Part model, mm, in its own coordinate system. A direction names the side the tool comes from. Round coordinates to 2 decimals unless told otherwise and drop trailing zeros.
1) Saw through at A-A on z = 686. Count the separate pieces of the cut face and the enclosed holes in it, and give its area (3 significant figures).
2) Which spindle directions (+Z, -Z, +X, -X, +Y, -Y) get a long thin tool onto all of the face, cutting with end or side? Do faces 1 (the cylindrical face through (6.81, -15.137, 493)), 2 (the flat face through (11, 14, 0)), 3 (the flat face through (52, 20, 493)). Say none if no direction does.
3) Pull direction X, two halves, no side cores. Call faces 4 (the flat face through (28, -20, 493)), 5 (the cylindrical face through (-7.972, -8.594, 493)), 6 (the flat face through (20, 52, 493)), 7 (the cylindrical face through (-15, 6.45, 493)): +X half, -X half, draft (parallel to the pull), parting line (faces both ways), or undercut.
4) Flat gauge pins, fed straight in: pin 1 (7.5 mm diameter, centred on x = 11.5, z = 603, fed in from -Y); pin 2 (5 mm diameter, centred on x = 30, y = -4, fed in from +Z); pin 3 (1 mm diameter, centred on x = 6, z = 274, fed in from -Y); pin 4 (2 mm diameter, centred on x = 32.5, z = 486.5, fed in from +Y). Where does each tip first touch, or does it go through?
5) Drill centre lines: L1, parallel to X at y = 48, z = 777; L2, parallel to Y at x = -2.5, z = 74; L3, parallel to X at y = 14.5, z = 181.5. Where is each one in solid material? Low to high.
```python
from build123d import *

# Parameters (mm, degrees)
SKETCH_1_R      = 3.4
SKETCH_1_R_2    = 4.3
EXTRUDE_1_DEPTH = 1000


with BuildPart() as part:
    # Эскиз1 → Бобышка-Вытянуть1 (new body)
    with BuildSketch(Plane.XY):
        with BuildLine():
            Line((-20, 47.35), (-20, 60))
            Line((-20, 60), (-7.35, 60))
            Line((-7.35, 60), (-4.1, 60))
            Line((-4.1, 60), (-4.1, 56.4))
            Line((-4.1, 56.4), (-7.35, 56.4))
            Line((-7.35, 56.4), (-7.35, 49.4))
            ThreePointArc((-7.35, 49.4), (0, 45.918928476), (7.35, 49.4))
            Line((7.35, 49.4), (7.35, 56.4))
            Line((7.35, 56.4), (4.1, 56.4))
            Line((4.1, 56.4), (4.1, 60))
            Line((4.1, 60), (7.35, 60))
            Line((7.35, 60), (20, 60))
            Line((20, 60), (20, 47.35))
            Line((20, 47.35), (20, 44.1))
            Line((20, 44.1), (16.4, 44.1))
            Line((16.4, 44.1), (16.4, 47.35))
            Line((16.4, 47.35), (9.4, 47.35))
            ThreePointArc((9.4, 47.35), (5.918928476, 40), (9.4, 32.65))
            Line((9.4, 32.65), (16.4, 32.65))
            Line((16.4, 32.65), (16.4, 35.9))
            Line((16.4, 35.9), (20, 35.9))
            Line((20, 35.9), (20, 32.65))
            Line((20, 32.65), (20, 29.1))
            ThreePointArc((20, 29.1), (13.565328291, 13.565328291), (29.1, 20))
            Line((29.1, 20), (32.65, 20))
            Line((32.65, 20), (35.9, 20))
            Line((35.9, 20), (35.9, 16.4))
            Line((35.9, 16.4), (32.65, 16.4))
            Line((32.65, 16.4), (32.65, 9.4))
            ThreePointArc((32.65, 9.4), (40, 5.918928476), (47.35, 9.4))
            Line((47.35, 9.4), (47.35, 16.4))
            Line((47.35, 16.4), (44.1, 16.4))
            Line((44.1, 16.4), (44.1, 20))
            Line((44.1, 20), (47.35, 20))
            Line((47.35, 20), (60, 20))
            Line((60, 20), (60, 7.35))
            Line((60, 7.35), (60, 4.1))
            Line((60, 4.1), (56.4, 4.1))
            Line((56.4, 4.1), (56.4, 7.35))
            Line((56.4, 7.35), (49.4, 7.35))
            ThreePointArc((49.4, 7.35), (45.918928476, 0), (49.4, -7.35))
            Line((49.4, -7.35), (56.4, -7.35))
            Line((56.4, -7.35), (56.4, -4.1))
            Line((56.4, -4.1), (60, -4.1))
            Line((60, -4.1), (60, -7.35))
            Line((60, -7.35), (60, -20))
            Line((60, -20), (47.35, -20))
            Line((47.35, -20), (44.1, -20))
            Line((44.1, -20), (44.1, -16.4))
            Line((44.1, -16.4), (47.35, -16.4))
            Line((47.35, -16.4), (47.35, -9.4))
            ThreePointArc((47.35, -9.4), (40, -5.918928476), (32.65, -9.4))
            Line((32.65, -9.4), (32.65, -16.4))
            Line((32.65, -16.4), (35.9, -16.4))
            Line((35.9, -16.4), (35.9, -20))
            Line((35.9, -20), (32.65, -20))
            Line((32.65, -20), (20, -20))
            ThreePointArc((20, -20), (-8.284271247, -8.284271247), (-20, 20))
            Line((-20, 20), (-20, 32.65))
            Line((-20, 32.65), (-20, 35.9))
            Line((-20, 35.9), (-16.4, 35.9))
            Line((-16.4, 35.9), (-16.4, 32.65))
            Line((-16.4, 32.65), (-9.4, 32.65))
            ThreePointArc((-9.4, 32.65), (-5.918928476, 40), (-9.4, 47.35))
            Line((-9.4, 47.35), (-16.4, 47.35))
            Line((-16.4, 47.35), (-16.4, 44.1))
            Line((-16.4, 44.1), (-20, 44.1))
            Line((-20, 44.1), (-20, 47.35))
        make_face()
        with Locations((0, 40)):
            Circle(SKETCH_1_R, mode=Mode.SUBTRACT)
        with Locations((-13.5, 53.5)):
            Circle(SKETCH_1_R_2, mode=Mode.SUBTRACT)
        with Locations((13.5, 53.5)):
            Circle(SKETCH_1_R_2, mode=Mode.SUBTRACT)
        with Locations((40, 0)):
            Circle(SKETCH_1_R, mode=Mode.SUBTRACT)
        with Locations((53.5, 13.5)):
            Circle(SKETCH_1_R_2, mode=Mode.SUBTRACT)
        with Locations((53.5, -13.5)):
            Circle(SKETCH_1_R_2, mode=Mode.SUBTRACT)
        with BuildLine():
            Line((-16.5, 30.25), (-8.9, 30.25))
            ThreePointArc((-8.9, 30.25), (-6.700552447, 32.329425303), (-4.963344147, 34.808071396))
            ThreePointArc((-4.963344147, 34.808071396), (-4.307204214, 35.295967153), (-3.506330333, 35.131155415))
            ThreePointArc((-3.506330333, 35.131155415), (-0.007297066, 34.000004437), (3.494477209, 35.122641182))
            ThreePointArc((3.494477209, 35.122641182), (4.300644961, 35.284393495), (4.955538691, 34.787217011))
            ThreePointArc((4.955538691, 34.787217011), (7.479168525, 31.392379507), (10.850248541, 28.837100905))
            ThreePointArc((10.850248541, 28.837100905), (11.347237818, 28.148388812), (11.135414137, 27.32592093))
            ThreePointArc((11.135414137, 27.32592093), (8.507881499, 20.42569046), (10.617718004, 13.349978606))
            ThreePointArc((10.617718004, 13.349978606), (10.798307809, 12.687415803), (10.508974176, 12.064609095))
            Line((10.508974176, 12.064609095), (3.943940688, 5.499575606))
            ThreePointArc((3.943940688, 5.499575606), (3.388591606, 5.218264662), (2.774429063, 5.320013475))
            ThreePointArc((2.774429063, 5.320013475), (-4.242640687, 4.242640687), (-5.320013475, -2.774429063))
            ThreePointArc((-5.320013475, -2.774429063), (-5.218264662, -3.388591606), (-5.499575606, -3.943940688))
            Line((-5.499575606, -3.943940688), (-6.633181618, -5.0775467))
            ThreePointArc((-6.633181618, -5.0775467), (-7.373462786, -5.369889497), (-8.092728627, -5.029100457))
            ThreePointArc((-8.092728627, -5.029100457), (-15.070519309, 6.630700987), (-17.5, 20))
            Line((-17.5, 20), (-17.5, 29.25))
            ThreePointArc((-17.5, 29.25), (-17.207106781, 29.957106781), (-16.5, 30.25))
        make_face(mode=Mode.SUBTRACT)
        with BuildLine():
            Line((29.25, -17.5), (20, -17.5))
            ThreePointArc((20, -17.5), (6.630700987, -15.070519309), (-5.029100457, -8.092728627))
            ThreePointArc((-5.029100457, -8.092728627), (-5.369889497, -7.373462786), (-5.0775467, -6.633181618))
            Line((-5.0775467, -6.633181618), (-3.943940688, -5.499575606))
            ThreePointArc((-3.943940688, -5.499575606), (-3.388591606, -5.218264662), (-2.774429063, -5.320013475))
            ThreePointArc((-2.774429063, -5.320013475), (-1.428271534, -5.827524382), (0, -6))
            ThreePointArc((0, -6), (1.3, -4.7), (0, -3.4))
            ThreePointArc((0, -3.4), (-2.404163056, 2.404163056), (3.4, 0))
            ThreePointArc((3.4, 0), (4.7, -1.3), (6, 0))
            ThreePointArc((6, 0), (5.827524382, 1.428271534), (5.320013475, 2.774429063))
            ThreePointArc((5.320013475, 2.774429063), (5.218264662, 3.388591606), (5.499575606, 3.943940688))
            Line((5.499575606, 3.943940688), (12.064609095, 10.508974176))
            ThreePointArc((12.064609095, 10.508974176), (12.687415803, 10.798307809), (13.349978606, 10.617718004))
            ThreePointArc((13.349978606, 10.617718004), (20.42569046, 8.507881499), (27.32592093, 11.135414137))
            ThreePointArc((27.32592093, 11.135414137), (28.148388812, 11.347237818), (28.837100905, 10.850248541))
            ThreePointArc((28.837100905, 10.850248541), (31.392379507, 7.479168525), (34.787217011, 4.955538691))
            ThreePointArc((34.787217011, 4.955538691), (35.284393495, 4.300644961), (35.122641182, 3.494477209))
            ThreePointArc((35.122641182, 3.494477209), (34.000004437, -0.007297066), (35.131155415, -3.506330333))
            ThreePointArc((35.131155415, -3.506330333), (35.295967153, -4.307204214), (34.808071396, -4.963344147))
            ThreePointArc((34.808071396, -4.963344147), (32.329425303, -6.700552447), (30.25, -8.9))
            Line((30.25, -8.9), (30.25, -16.5))
            ThreePointArc((30.25, -16.5), (29.957106781, -17.207106781), (29.25, -17.5))
        make_face(mode=Mode.SUBTRACT)
    extrude(amount=EXTRUDE_1_DEPTH)


solid = part.part
```
Completed:
1. separate pieces: 1
1. enclosed holes: 8
1. area: 1,370 mm2
2. face 1: +Z, -Z
2. face 2: -Z, +X, -X, +Y, -Y
2. face 3: +Z, -Z, +X, +Y
3. face 4: draft
3. face 5: -X half
3. face 6: +X half
3. face 7: undercut
4. pin 1: stops at y = -19.72
4. pin 2: passes through
4. pin 3: stops at y = -17.65
4. pin 4: stops at y = 20
5. L1: x = -20 to -5.93, 5.93 to 20
5. L2: y = -13.07 to -10.12, -5.45 to -2.3, 2.3 to 5.45, 34.55 to 37.7, 42.3 to 46.25
5. L3: x = -19.62 to -17.1, 9.9 to 12.75, 27.25 to 32.65, 47.35 to 49.32, 57.68 to 60
